Source: CAD feature listing. Evaluate the final solid. Frame: model axes, mm. Give positions to 0.01 mm unless a question says otherwise; leave off trailing zeros. Order: outer loops, then holes, each group sorted by start corner. A loop starts at its lowest first (then second) coordinate and runs counter-clockwise, first axis right, second up. Notation, with made-up numbers: M 31.25,-22.75 L 86.25,-22.75 A17 ccw 86.25,-9.75 Z; hole C 8.5,-23.5 d11. An arc over 180 degrees is marked long. Answer in a Markdown table with one row per item. Add a question column.
(1) Section query B-B, the plane z = 76. Return loops of the section in (x, y), plus the area to 3 significant figures.
(2) Mould query, pull axis Y, two halves, no side actions, for faces 1 (the face through (90, 127, 50)), 2 (the face through (72.58, 53.36, 50.09)), 3 (the face through (123, 64, 0)). Classes: pulls with the +Y half, pulls with the -Y half, needs draft (parallel to the pull), parting line crosses it, or undercut.
(3) Section query A-A, the plane y = 92. Return loops of the section in (x, z).
(4) Material intervals for line 1 along X through (y, z) = (71, 7.5); line 2 along X through (y, z) = (48, 4.5); line 3 along Y through (x, z) = (103.5, 87), sorted ascending.
(5) Section query C-C, the plane y = 63. Return loops of the section in (x, z).
from build123d import *

# Parameters (mm, degrees)
F0_R     = 26.300006
F1_DEPTH = 101.6


with BuildPart() as f1:
    # F0 (on Top) → F1 (new body)
    with BuildSketch(Plane.XY):
        with BuildLine():
            Line((0, 127), (0, 0))
            Line((0, 0), (203.2, 0))
            Line((203.2, 0), (203.2, 101.6))
            ThreePointArc((203.2, 101.6), (195.760512, 119.560512), (177.8, 127))
            Line((177.8, 127), (0, 127))
        make_face()
        with Locations((93.450926, 69.365256)):
            Circle(F0_R, mode=Mode.SUBTRACT)
    extrude(amount=F1_DEPTH)


solid = f1.part
Values follow:
| question | item | result |
|---|---|---|
| 1 | outline | M 0,0 L 203.2,0 L 203.2,101.6 A25.4 ccw 177.8,127 L 0,127 Z; hole C 93.45,69.37 d52.6 |
| 1 | area | 23,500 mm² |
| 2 | face 1 | pulls with the +Y half |
| 2 | face 2 | undercut |
| 2 | face 3 | needs draft |
| 3 | outline | M 0,0 L 80.06,0 L 80.06,101.6 L 0,101.6 Z; M 106.84,0 L 203.2,0 L 203.2,101.6 L 106.84,101.6 Z |
| 4 | line 1 | x = 0 to 67.2, 119.7 to 203.2 |
| 4 | line 2 | x = 0 to 78.11, 108.79 to 203.2 |
| 4 | line 3 | y = 0 to 45.06, 93.67 to 127 |
| 5 | outline | M 0,0 L 67.93,0 L 67.93,101.6 L 0,101.6 Z; M 118.97,0 L 203.2,0 L 203.2,101.6 L 118.97,101.6 Z |
